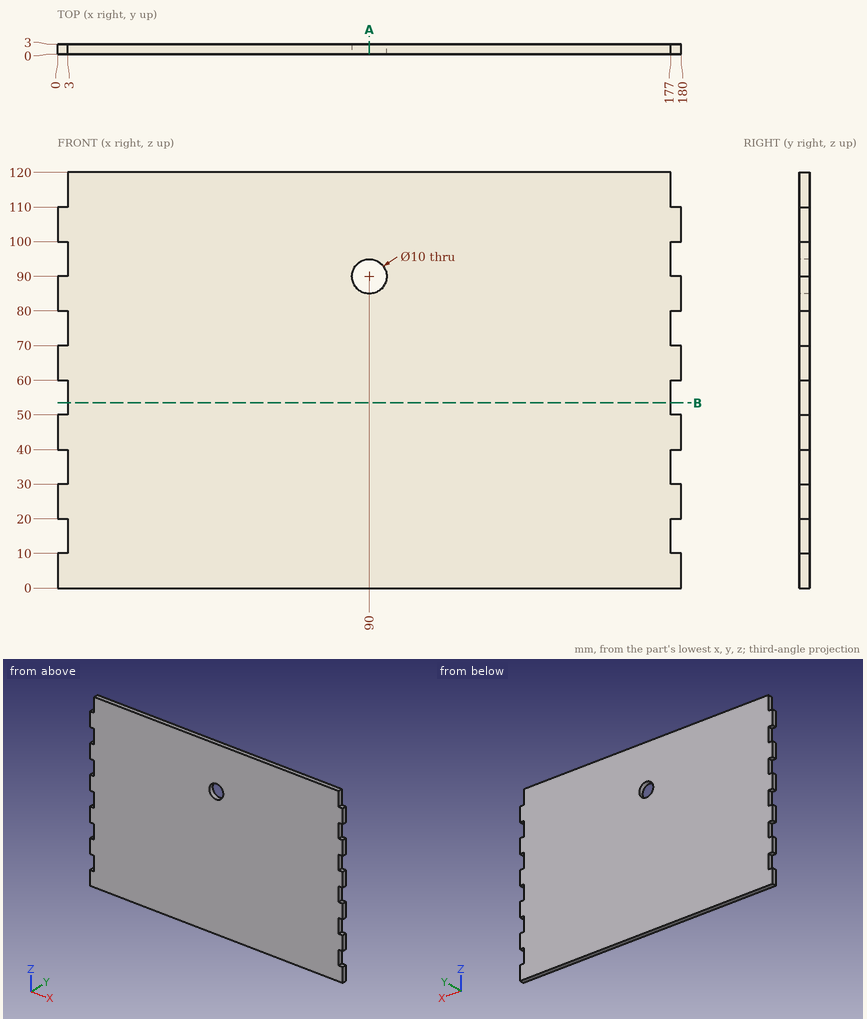
Verification items for this drawing (mm, ordinates from the low corner). Give positions to 0.01 mm unless a question says otherwise; leave off trailing zeros. Loops run counter-clockwise (first coordinate to the right, second up) from the corner with the lowest first, then second, coordinate; pieces in that order, holes last. Notation, with made-up numbers: M 43.25,-29.5 L 54.25,-29.5 A19 cw 54.25,-24.5 Z; hole C -9.5,-38 d6. An arc over 180 degrees is marked long. Return JSON: item names as keys, results as strings. Group by question number.
1. Thickness scan on L1, parallel to X at y = 1.95, z = 110.5; L2, parallel to Z at x = 90, y = 1.6; L3, parallel to X at y = 0.8, z = 92. Record the ranges inside material, lowest first.
2. Go/stop test with flat-tipped pins: pin 1 (0.9 mm diameter, centred on x = 179, y = 2, fed in from +Z); pin 2 (1.5 mm diameter, centred on y = 1, z = 14.5, fed in from -X); pin 3 (1.5 mm diameter, centred on y = 2, z = 76, fed in from +X). Record where each tip stops, or that it passes through.
3. Cross-section at A-A on x = 90. Record the boundary of the cut face in (y, z).
4. Cross-section at B-B on z = 53.5. Record the boundary of the cut face in (x, y).
Return value:
{
 "1": {"L1": "3 to 177", "L2": "0 to 85, 95 to 120", "L3": "3 to 85.42, 94.58 to 177"},
 "2": {"pin 1": "z = 110", "pin 2": "x = 3", "pin 3": "x = 177"},
 "3": {"outline": "M 0,0 L 3,0 L 3,85 L 0,85 Z; M 0,95 L 3,95 L 3,120 L 0,120 Z"},
 "4": {"outline": "M 3,0 L 177,0 L 177,3 L 3,3 Z"}
}
